Build history of the part. All positions in model axes, mm. A direction names the side the tool comes from. Round coordinates to 2 decimals unless told otherwise and drop trailing zeros. Write each loop counter-clockwise with the first axis right and the second up, starting at its lowest first coordinate (ties: lowest second). Pieces come first, ordered by that corner, then holes. Notation, with made-up numbers: (31.25, -18.5) -> (36.25, -18.5) arc R8 cw to (36.25, -5.5) -> close; hole circle Ø4 at (64.25, 46.5). An arc over 180 degrees is marked (long way). Answer as CSV lines item,"result".
from build123d import *

# Parameters (mm, degrees)
SKETCH1_R           = 25
BOSS_EXTRUDE1_DEPTH = 2
SKETCH2_R           = 3.772478216
SKETCH2_R_2         = 3.395230394
BOSS_EXTRUDE2_DEPTH = 10
SKETCH3_W           = 11.380817266
SKETCH3_H           = 5.470093412
BOSS_EXTRUDE3_DEPTH = 5
SKETCH4_R           = 1.574884911
SKETCH4_R_2         = 1.887966751
CUT_EXTRUDE1_DEPTH  = 5


with BuildPart() as part:
    # Sketch1 → Boss-Extrude1 (new body)
    with BuildSketch(Plane.XY):
        Circle(SKETCH1_R)
    extrude(amount=BOSS_EXTRUDE1_DEPTH)

    # Sketch2 → Boss-Extrude2 (add)
    with BuildSketch(Plane.XY.offset(2)):
        with Locations((0, 14.712665041)):
            Circle(SKETCH2_R)
        with Locations((18.611146521, 0)):
            Circle(SKETCH2_R_2)
    extrude(amount=BOSS_EXTRUDE2_DEPTH)

    # Sketch3 → Boss-Extrude3 (add)
    with BuildSketch(Plane.XY.offset(2)):
        Rectangle(SKETCH3_W, SKETCH3_H)
    extrude(amount=BOSS_EXTRUDE3_DEPTH)

    # Sketch4 → Cut-Extrude1 (cut)
    with BuildSketch(Plane.XY.offset(2)):
        with Locations((-14.865882925, -13.379294632)):
            Circle(SKETCH4_R)
        with Locations((14.865882925, 13.379294632)):
            Circle(SKETCH4_R_2)
    extrude(amount=-CUT_EXTRUDE1_DEPTH, mode=Mode.SUBTRACT)


solid = part.part
1. Mould opens along Y. For faces 1 (the flat face through (5.69, 0, 4)), 2 (the flat face through (0, 2.735, 4)), 3 (the cylindrical face through (23.846, 7.509, 0.986)) say: +Y half, -Y half, draft (parallel to the pull), parting line (faces both ways), or undercut.
Results found:
face 1,"draft"
face 2,"undercut"
face 3,"parting line"
2. Which spindle directions (+Z, -Z, +X, -X, +Y, -Y) get a long thin tool onto all of the face, cutting with end or side? Do faces 4 (the flat face through (-5.69, 0, 4)), 5 (the flat face through (0, -2.735, 4)), 6 (the cylindrical face through (-0.82, 11.03, 6.93)). Say none if no direction does.
Results found:
face 4,"+Z, -X, +Y, -Y"
face 5,"+Z, -X, -Y"
face 6,"+Z"
3. Probe line 1 along Z through (x, y) = (0.5, 21); line 2 along X through (y, z) = (2.5, 4.25); line 3 along X through (y, z) = (15, 6). List the from-to ranges inside material, lowest first.
Results found:
line 1,"z = 0 to 2"
line 2,"x = -5.69 to 5.69, 16.31 to 20.91"
line 3,"x = -3.76 to 3.76"
4. Cut at C-C, the plane z = 4. Write the cut outline in (x, y).
Results found:
outline,"(-5.69, -2.74) -> (5.69, -2.74) -> (5.69, 2.74) -> (-5.69, 2.74) -> close; circle Ø7.54 at (0, 14.71); circle Ø6.79 at (18.61, 0)"
5. Cut at B-B, the plane y = -12.5. Write the cut outline in (x, z).
Results found:
outline,"(-21.65, 0) -> (-16.17, 0) -> (-16.17, 2) -> (-21.65, 2) -> close; (-13.56, 0) -> (21.65, 0) -> (21.65, 2) -> (-13.56, 2) -> close"
6. Cut at D-D, the plane x = 0. Write the cut outline in (y, z), then the cut area to 3 significant figures.
Results found:
outline,"(-25, 0) -> (25, 0) -> (25, 2) -> (18.49, 2) -> (18.49, 12) -> (10.94, 12) -> (10.94, 2) -> (2.74, 2) -> (2.74, 7) -> (-2.74, 7) -> (-2.74, 2) -> (-25, 2) -> close"
area,"203 mm2"
7. Drop flat-ended pins along their axis: pin 1 Ø8 at (x, y) = (-10.5, 5) entering from +Z; pin 2 Ø5.5 at (x, z) = (-2, 5.5) entering from +Y; pin 3 Ø6 at (x, y) = (0.5, 1.5) entering from +Z; pin 4 Ø2.5 at (x, y) = (-14.87, -13.38) entering from -Z. Give the stop position or say it passes through.
Results found:
pin 1,"stops at z = 2"
pin 2,"stops at y = 18.49"
pin 3,"stops at z = 7"
pin 4,"passes through"
8. Cut at A-A, the plane x = 16. Write the cut outline in (y, z).
Results found:
outline,"(-19.21, 0) -> (11.87, 0) -> (11.87, 2) -> (2.17, 2) -> (2.17, 12) -> (-2.17, 12) -> (-2.17, 2) -> (-19.21, 2) -> close; (14.89, 0) -> (19.21, 0) -> (19.21, 2) -> (14.89, 2) -> close"
